```python
from build123d import *

# Parameters (mm, degrees)
SKETCH1_W                                         = 1.6002
SKETCH1_H                                         = 11.95
BOSS_EXTRUDE1_DEPTH                               = 23.685439
CUT_EXTRUDE1_DEPTH                                = 10
CSK_FOR_0_FLAT_HEAD_SOCKET_CAP_SCREW1_D           = 1.778
CSK_FOR_0_FLAT_HEAD_SOCKET_CAP_SCREW1_DEPTH       = 3
CSK_FOR_0_FLAT_HEAD_SOCKET_CAP_SCREW1_CSINK_D     = 3.5052
CSK_FOR_0_FLAT_HEAD_SOCKET_CAP_SCREW1_CSINK_ANGLE = 82
CSK_FOR_0_FLAT_HEAD_SOCKET_CAP_SCREW1_TIP         = 0.53416509


with BuildPart() as part:
    # Sketch1 → Boss-Extrude1 (new body)
    with BuildSketch(Plane.XY):
        with Locations((-2.5501, 9.975)):
            Rectangle(SKETCH1_W, SKETCH1_H)
    extrude(amount=BOSS_EXTRUDE1_DEPTH)

    # Sketch2 → Cut-Extrude1 (cut)
    with BuildSketch(Plane(origin=(-1.75, 0, 0), x_dir=(0, 0, -1), z_dir=(1, 0, 0))):
        with BuildLine():
            Line((-22.411068255, 4), (-1.27437031, 4))
            ThreePointArc((-1.27437031, 4), (-11.842719282, 11.3), (-22.411068255, 4))
        make_face()
    extrude(amount=-CUT_EXTRUDE1_DEPTH, mode=Mode.SUBTRACT)

    # CSK for #0 Flat Head Socket Cap Screw1
    with Locations(Plane.ZY.offset(3.3502)):
        with Locations((11.842719282, 13.95)):
            CounterSinkHole(CSK_FOR_0_FLAT_HEAD_SOCKET_CAP_SCREW1_D / 2, CSK_FOR_0_FLAT_HEAD_SOCKET_CAP_SCREW1_CSINK_D / 2, depth=CSK_FOR_0_FLAT_HEAD_SOCKET_CAP_SCREW1_DEPTH, counter_sink_angle=CSK_FOR_0_FLAT_HEAD_SOCKET_CAP_SCREW1_CSINK_ANGLE)
            with Locations((0, 0, -(CSK_FOR_0_FLAT_HEAD_SOCKET_CAP_SCREW1_DEPTH + CSK_FOR_0_FLAT_HEAD_SOCKET_CAP_SCREW1_TIP / 2))):  # 118° drill point
                Cone(0, CSK_FOR_0_FLAT_HEAD_SOCKET_CAP_SCREW1_D / 2, CSK_FOR_0_FLAT_HEAD_SOCKET_CAP_SCREW1_TIP, mode=Mode.SUBTRACT)


solid = part.part
```
The listing builds one solid part. Answer for the finished solid, in the listing's coordinates (mm). Give positions to 0.01 mm unless a question says otherwise; leave off trailing zeros. Order: outer loops, then holes, each group sorted by start corner. A loop starts at its lowest first (then second) coordinate and runs counter-clockwise, first axis right, second up. Notation, with made-up numbers: (-5, -36) -> (-1, -36) arc R20 ccw to (-1, -10) -> close; hole circle Ø4 at (44, 69.5). An arc over 180 degrees is marked (long way). Answer as CSV lines item,"result". Start each with the question number.
Q1. A cutting plane is placed at A-A (y = 13.95). Determine the outline of the cut face in (x, z), then the cut area to 3 significant figures.
Q2. Given pin 1 (3 mm diameter, centred on y = 6, z = 17, fed in from -X), flat-ended and moving along its own axis, determine where the tip first touches the part or whether it passes through.
Q3. Find the intervals of material crossed by L1, parallel to Z at x = -2.2, y = 13.95; L2, parallel to Y at x = -2.75, z = 12; L3, parallel to Z at x = -3.15, y = 7, in increasing order.
Q4. A cutting plane is placed at C-C (y = 6.5). Determine the outline of the cut face in (x, z), then the cut area to 3 significant figures.
Q5. A cutting plane is placed at D-D (z = 9). Determine the outline of the cut face in (x, y), then the cut area to 3 significant figures.
Q6. Determine the mould class of faces 1 (the cylindrical face through (-2.5, 11.3, 11.7)), 2 (the cylindrical face through (-2.05, 13.99, 12.73)), 3 (the flat face through (-3.35, 11.2, 9)) for opening direction Y: pulls with the +Y half, pulls with the -Y half, needs draft (parallel to the pull), parting line crosses it, or undercut.
Q7. A cutting plane is placed at B-B (x = -2). Determine the outline of the cut face in (y, z), then the cut area to 3 significant figures.
Results found:
1,outline,"(-3.35, 0) -> (-1.75, 0) -> (-1.75, 10.95) -> (-2.36, 10.95) -> (-3.35, 10.09) -> close; (-3.35, 13.6) -> (-2.36, 12.73) -> (-1.75, 12.73) -> (-1.75, 23.69) -> (-3.35, 23.69) -> close"
1,area,"34.2 mm2"
2,pin 1,"through"
3,L1,"0 to 10.95, 12.73 to 23.69"
3,L2,"11.3 to 12.73, 15.17 to 15.95"
3,L3,"0 to 2.97, 20.71 to 23.69"
4,outline,"(-3.35, 0) -> (-1.75, 0) -> (-1.75, 2.6) -> (-3.35, 2.6) -> close; (-3.35, 21.09) -> (-1.75, 21.09) -> (-1.75, 23.69) -> (-3.35, 23.69) -> close"
4,area,"8.32 mm2"
5,outline,"(-3.35, 10.94) -> (-1.75, 10.94) -> (-1.75, 15.95) -> (-3.35, 15.95) -> close"
5,area,"8.02 mm2"
6,face 1,"pulls with the -Y half"
6,face 2,"undercut"
6,face 3,"needs draft"
7,outline,"(4, 0) -> (15.95, 0) -> (15.95, 23.69) -> (4, 23.69) -> (4, 22.41) arc R11.3 cw to (4, 1.27) -> close; hole circle Ø1.78 at (13.95, 11.84)"
7,area,"168 mm2"
